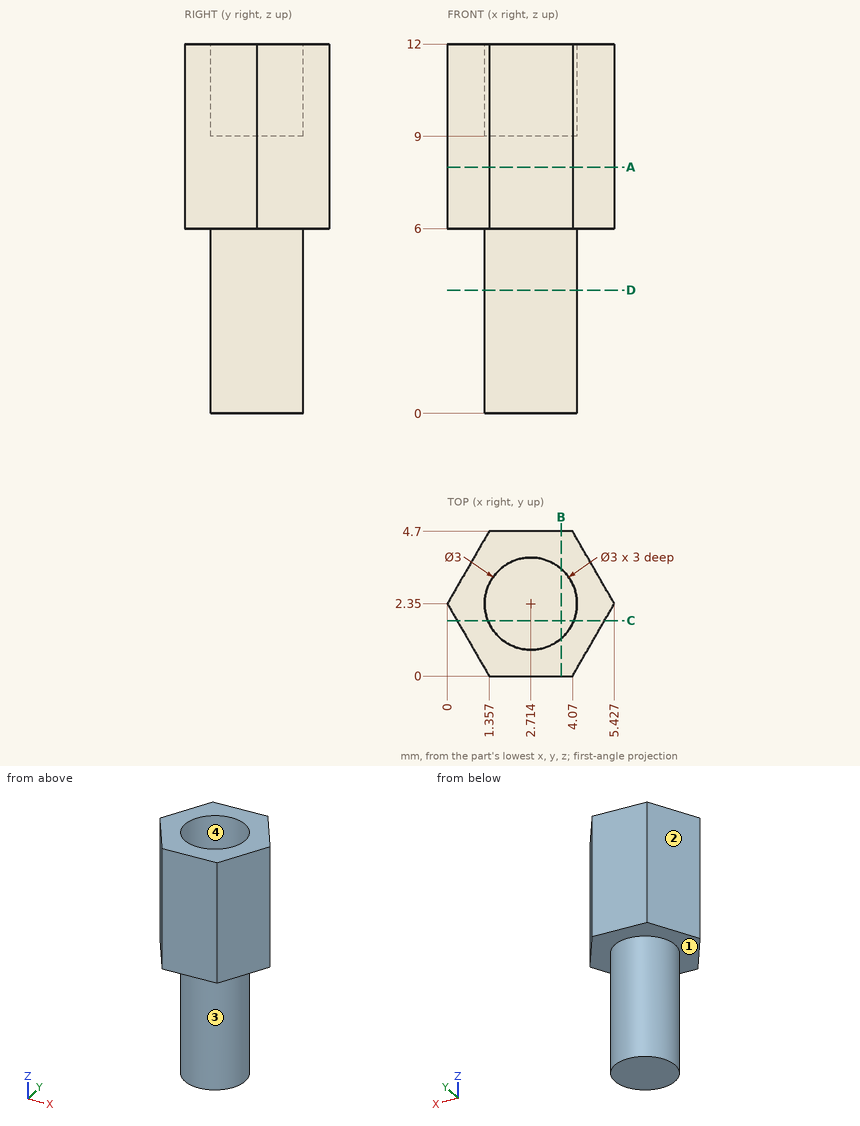
The figure shows three views and two pictorial views of one solid part (mm, origin at its lowest corner). Answer the questions. Coordinates: 2 decimals unless noted, no trailing zeros. Loops run counter-clockwise (first coordinate to the right, second up) from the corner with the lowest first, then second, coordinate; pieces in that order, holes last. Notation, with made-up numbers: (83.25, 16.5) -> (92.25, 16.5) arc R11 cw to (92.25, 21.5) -> close; hole circle Ø8 at (41.5, -8). An arc over 180 degrees is marked (long way). Return JSON: item names as keys, results as strings. Group by question number.
(1) Find the intervals of material crossed by probe 1 along Z at (x, y) = (4.4, 1.3); probe 2 along Z at (x, y) = (3.6, 1.9); probe 3 along Y at (x, z) = (2.7, 2), in increasing order. Write a range as from..to.
(2) A cutting plane is placed at D-D on z = 4. Write down the section's boundary in (x, y).
(3) Given pin 1 Ø0.9 at (x, y) = (3, 2) entering from +Z, flat-ended and moving along its own axis, determine where the tip first touches the part or whether it passes through.
(4) A cutting plane is placed at A-A on z = 8. Write down the section's boundary in (x, y).
(5) A cutting plane is placed at B-B on x = 3.7. Write down the section's boundary in (y, z).
(6) Determine the mould class of the marked faces 1, 2, 3 and 4 for opening direction X: released by +X, released by -X, zero draft, split by the parting line, or undercut.
(7) A cutting plane is placed at C-C on y = 1.8. Write down the section's boundary in (x, z).
The answers:
{
 "1": {"probe 1": "z = 6..12", "probe 2": "z = 0..9", "probe 3": "y = 0.85..3.85"},
 "2": {"outline": "circle Ø3 at (2.71, 2.35)"},
 "3": {"pin 1": "stops at z = 9"},
 "4": {"outline": "(0, 2.35) -> (1.36, 0) -> (4.07, 0) -> (5.43, 2.35) -> (4.07, 4.7) -> (1.36, 4.7) -> close"},
 "5": {"outline": "(0, 6) -> (1.22, 6) -> (1.22, 0) -> (3.48, 0) -> (3.48, 6) -> (4.7, 6) -> (4.7, 12) -> (3.48, 12) -> (3.48, 9) -> (1.22, 9) -> (1.22, 12) -> (0, 12) -> close"},
 "6": {"face 1": "zero draft", "face 2": "released by -X", "face 3": "split by the parting line", "face 4": "undercut"},
 "7": {"outline": "(0.32, 6) -> (1.32, 6) -> (1.32, 0) -> (4.11, 0) -> (4.11, 6) -> (5.11, 6) -> (5.11, 12) -> (4.11, 12) -> (4.11, 9) -> (1.32, 9) -> (1.32, 12) -> (0.32, 12) -> close"}
}
